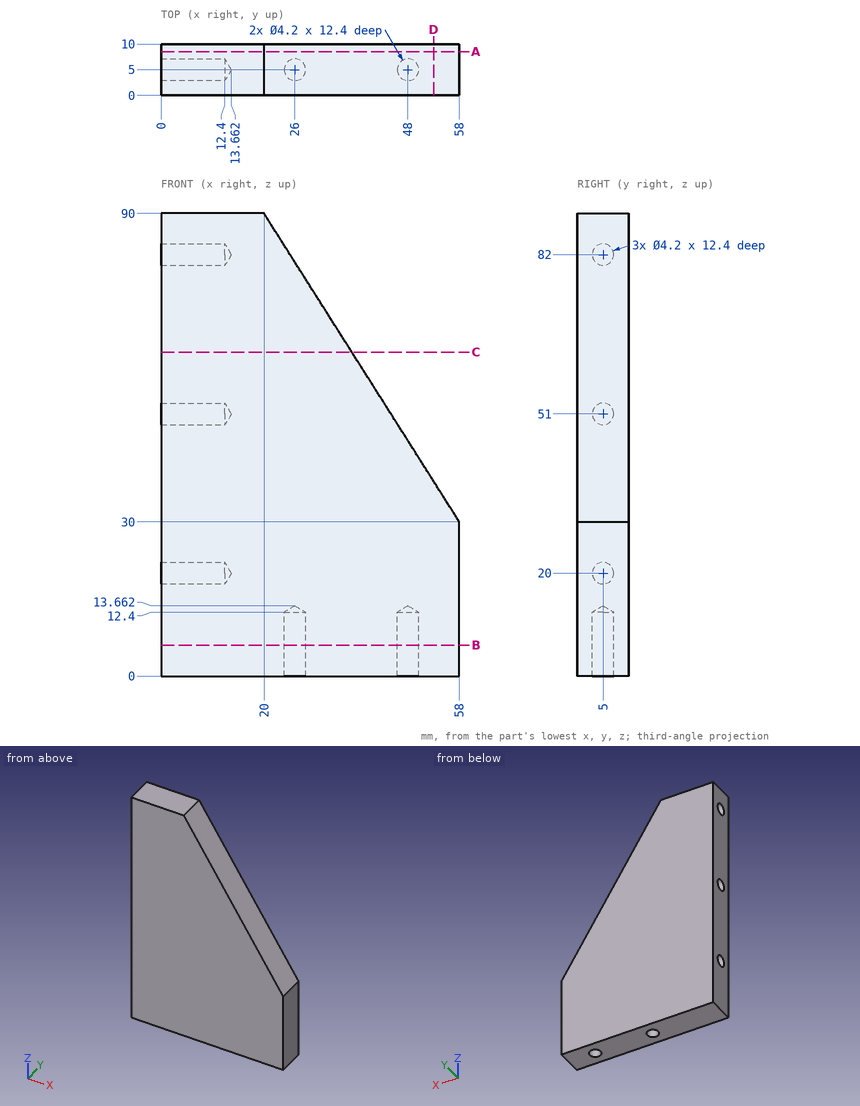
Check sheet for the drawn part. Datum: minimum x, y, z corner. Units: mm. Coordinates: 2 decimals unless noted, no trailing zeros. Loops run counter-clockwise (first coordinate to the right, second up) from the corner with the lowest first, then second, coordinate; pieces in that order, holes last. Notation, with made-up numbers: (32.25, -15.5) -> (44.25, -15.5) arc R22 cw to (44.25, -2.5) -> close; hole circle Ø1 at (-37, 56). An arc over 180 degrees is marked (long way). Answer in a Markdown table with one row per item.
1. Sectioned sample at D-D, the plane x = 53. Record the boundary of the cut face in (y, z) (1 decimal).
Check values:
| item | result |
|---|---|
| outline | (0, 0) -> (10, 0) -> (10, 37.9) -> (0, 37.9) -> close |
2. Sectioned sample at B-B, the plane z = 6. Record the boundary of the cut face in (x, y), then the cut area to 3 significant figures.
Check values:
| item | result |
|---|---|
| outline | (0, 0) -> (58, 0) -> (58, 10) -> (0, 10) -> close; hole circle Ø4.2 at (26, 5); hole circle Ø4.2 at (48, 5) |
| area | 552 mm2 |
3. Go/stop test with flat-tipped pins: pin 1 (1.5 mm diameter, centred on y = 4, z = 39.5, fed in from +X); pin 2 (5 mm diameter, centred on y = 5, z = 82, fed in from +X); pin 3 (4 mm diameter, centred on x = 48, y = 5, fed in from +Z). Record where each tip stops, or that it passes through.
Check values:
| item | result |
|---|---|
| pin 1 | stops at x = 52.46 |
| pin 2 | stops at x = 26.65 |
| pin 3 | stops at z = 48.95 |
4. Material ranges on line 1 along Z through (x, y) = (10.25, 5); line 2 along Y through (x, z) = (5.5, 51); line 3 along Z through (x, y) = (6.5, 6.5), recorded low to high. Write a range as [from, to].
Check values:
| item | result |
|---|---|
| line 1 | z = [0, 17.9], [22.1, 48.9], [53.1, 79.9], [84.1, 90] |
| line 2 | y = [0, 2.9], [7.1, 10] |
| line 3 | z = [0, 18.53], [21.47, 49.53], [52.47, 80.53], [83.47, 90] |
5. Sectioned sample at A-A, the plane y = 8.5. Record the boundary of the cut face in (x, z), then the cut area to 3 significant figures.
Check values:
| item | result |
|---|---|
| outline | (0, 0) -> (58, 0) -> (58, 30) -> (20, 90) -> (0, 90) -> close |
| area | 4,080 mm2 |
6. Sectioned sample at C-C, the plane z = 63. Record the boundary of the cut face in (x, y).
Check values:
| item | result |
|---|---|
| outline | (0, 0) -> (37.1, 0) -> (37.1, 10) -> (0, 10) -> close |
